Check sheet for the modelled part. Datum: model origin and axes. Units: mm. Face numbers are marked on the shaded views. A direction names the side the tool comes from. Give positions to 0.01 mm unless a question says otherwise; leave off trailing zeros. Order: outer loops, then holes, each group sorted by start corner. A loop starts at its lowest first (then second) coordinate and runs counter-clockwise, first axis right, second up.
```python
from build123d import *

# Parameters (mm, degrees)
SKETCH1_R           = 1.7272
BOSS_EXTRUDE1_DEPTH = 9.271
SKETCH2_R           = 3.429
BOSS_EXTRUDE2_DEPTH = 2.54
FILLET1_R           = 1.905
CUT_EXTRUDE1_DEPTH  = 1.905


with BuildPart() as part:
    # Sketch1 → Boss-Extrude1 (new body)
    with BuildSketch(Plane.XY):
        Circle(SKETCH1_R)
    extrude(amount=BOSS_EXTRUDE1_DEPTH)

    # Sketch2 → Boss-Extrude2 (add)
    with BuildSketch(Plane.XY.offset(9.271)):
        Circle(SKETCH2_R)
    extrude(amount=BOSS_EXTRUDE2_DEPTH)

    # Fillet1
    fillet1_edges = [part.edges().sort_by_distance(p)[0] for p in [
        (-3.429, 0, 11.811),
    ]]
    fillet(fillet1_edges, radius=FILLET1_R)

    # Sketch3 → Cut-Extrude1 (cut)
    with BuildSketch(Plane.XY.offset(11.811)):
        Polygon((-0.303567799, 0.303567799), (-0.303567799, 2.17637078), (0.303567799, 2.17637078), (0.303567799, 0.303567799), (2.17637078, 0.303567799), (2.17637078, -0.303567799), (0.303567799, -0.303567799), (0.303567799, -2.17637078), (-0.303567799, -2.17637078), (-0.303567799, -0.303567799), (-2.17637078, -0.303567799), (-2.17637078, 0.303567799), align=None)
    extrude(amount=-CUT_EXTRUDE1_DEPTH, mode=Mode.SUBTRACT)


solid = part.part
```
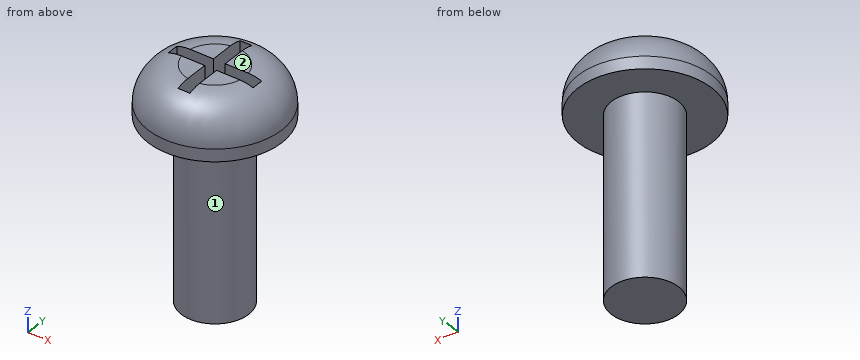
(1) Tool access check on the marked faces 1 and 2. Record the directions out of +Z, -Z, +X, -X, +Y, -Y that give a thin tool (end or side, any length) a straight path to the whole face; none if there is none.
(2) Sectioned sample at A-A (z = 4.5). Enter the section's corners in (x, y).
(3) Go/stop test with flat-tipped pins: P1, Ø2, axis at x = 1.5, z = 10.5, coming from the -Y side; P2, Ø0.9, axis at y = 1.5, z = 11, coming from the +X side; P3, Ø2, axis at y = 1, z = 11, coming from the -X side. Record where each tip stops, or that it passes through.
(4) Thickness scan on L1, parallel to Z at x = 1.75, y = 0.25; L2, parallel to Z at x = -1.5, y = -2; L3, parallel to Y at x = 1.5, z = 6. Record the ranges inside material, lowest first.
Values follow:
1. face 1: -Z
1. face 2: +Z, +X, -X, +Y, -Y
2. outline: circle Ø3.45 at (0, 0)
3. P1: stops at y = -3.37
3. P2: stops at x = 3.04
3. P3: stops at x = -3.38
4. L1: z = 9.27 to 9.91
4. L2: z = 9.27 to 11.54
4. L3: y = -0.86 to 0.86
